Design review of the part built by this model. Coordinates are the model's own, in mm. Face numbers are marked on the shaded views. Coordinates: 2 decimals unless noted, no trailing zeros. Write each loop counter-clockwise with the first axis right and the second up, starting at its lowest first coordinate (ties: lowest second). Pieces come first, ordered by that corner, then holes. Notation, with made-up numbers: M -9.75,51 L 35.25,51 A24 ccw 35.25,81 Z; hole C 14,24.25 d4. An arc over 180 degrees is marked long. Return JSON: item names as keys, results as strings. Group by question number.
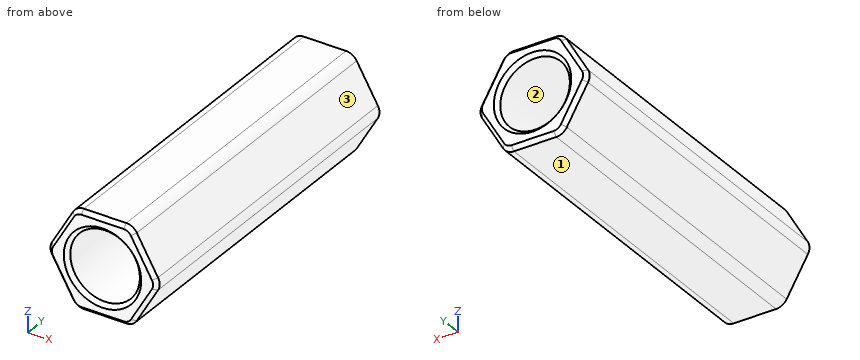
```python
from build123d import *

# Parameters (mm, degrees)
BOSS_EXTRUDE1_DEPTH   = 5.55625
F_4_40_TAPPED_HOLE1_D = 2.2606
FILLET1_R             = 0.396875
CHAMFER1_SIZE         = 0.127


with BuildPart() as part:
    # Sketch1 → Boss-Extrude1 (new body, symmetric)
    with BuildSketch(Plane(origin=(0, 0, 0), x_dir=(1, 0, 0), z_dir=(0, 1, 0))):
        Polygon((0.916543552, 1.5875), (-0.916543552, 1.5875), (-1.833087105, 0), (-0.916543552, -1.5875), (0.916543552, -1.5875), (1.833087105, 0), align=None)
    extrude(amount=BOSS_EXTRUDE1_DEPTH, both=True)

    # #4-40 Tapped Hole1 (through all)
    with Locations(Plane(origin=(0, 5.55625, 0), x_dir=(1, 0, 0), z_dir=(0, 1, 0))):
        with Locations((0, 0)):
            Hole(F_4_40_TAPPED_HOLE1_D / 2)

    # Fillet1
    fillet1_edges = [part.edges().sort_by_distance(p)[0] for p in [
        (1.833087105, 0, 0),
        (0.916543552, 0, 1.5875),
        (-0.916543552, 0, 1.5875),
        (-1.833087105, 0, 0),
        (-0.916543552, 0, -1.5875),
        (0.916543552, 0, -1.5875),
    ]]
    fillet(fillet1_edges, radius=FILLET1_R)

    # Chamfer1
    chamfer1_edges = [part.edges().sort_by_distance(p)[0] for p in [
        (1.1303, 5.55625, 0),
        (1.1303, -5.55625, 0),
        (-1.374815329, -5.55625, -0.79375),
        (-1.374815329, 5.55625, -0.79375),
        (1.374815329, -5.55625, -0.79375),
        (1.374815329, -5.55625, 0.79375),
        (0, -5.55625, 1.5875),
        (-1.374815329, -5.55625, 0.79375),
        (0, -5.55625, -1.5875),
        (-1.771690329, -5.55625, 0),
        (-0.885845164, -5.55625, 1.534328832),
        (0.885845164, -5.55625, 1.534328832),
        (1.771690329, -5.55625, 0),
        (0.885845164, -5.55625, -1.534328832),
        (-0.885845164, -5.55625, -1.534328832),
        (0, 5.55625, -1.5875),
        (1.374815329, 5.55625, -0.79375),
        (-1.374815329, 5.55625, 0.79375),
        (0, 5.55625, 1.5875),
        (1.374815329, 5.55625, 0.79375),
        (-1.771690329, 5.55625, 0),
        (-0.885845164, 5.55625, 1.534328832),
        (0.885845164, 5.55625, 1.534328832),
        (1.771690329, 5.55625, 0),
        (0.885845164, 5.55625, -1.534328832),
        (-0.885845164, 5.55625, -1.534328832),
    ]]
    chamfer(chamfer1_edges, length=CHAMFER1_SIZE)


solid = part.part
```
Item 1: The part is to be moulded in two halves that separate along Z. For the marked faces 1, 2 and 3, say which applies: pulls with the +Z half, pulls with the -Z half, needs draft (parallel to the pull), parting line crosses it, or undercut.
Item 2: Add section C-C (z = 0). Write out the cut boundary in (x, y).
Item 3: Add section A-A (x = 0). Write out the cut boundary in (y, z), plus the area to 3 significant figures.
Item 4: For pin 1 (1.5 mm diameter, centred on y = -4, z = 0.5, fed in from +X); pin 2 (1.5 mm diameter, centred on y = 1, z = -1, fed in from +X), all flat-tipped, find the tip position at first contact; note any pin that passes through.
Item 5: For line 1 (X direction, y = 0, z = 0); line 2 (Z direction, x = 0, y = -1); line 3 (X direction, y = 2.25, z = -0.9), list the stretches that pass through material, from the lowest coordinate up.
Item 6: Add section B-B (y = 1.75). Write out the cut boundary in (x, z), plus the area to 3 significant figures.
Geometry check:
{
 "1": {"face 1": "pulls with the -Z half", "face 2": "undercut", "face 3": "pulls with the +Z half"},
 "2": {"outline": "M -1.77,-5.43 L -1.64,-5.56 L -1.26,-5.56 L -1.13,-5.43 L -1.13,5.43 L -1.26,5.56 L -1.64,5.56 L -1.77,5.43 Z; M 1.13,-5.43 L 1.26,-5.56 L 1.64,-5.56 L 1.77,-5.43 L 1.77,5.43 L 1.64,5.56 L 1.26,5.56 L 1.13,5.43 Z"},
 "3": {"outline": "M -5.56,-1.46 L -5.43,-1.59 L 5.43,-1.59 L 5.56,-1.46 L 5.56,-1.26 L 5.43,-1.13 L -5.43,-1.13 L -5.56,-1.26 Z; M -5.56,1.26 L -5.43,1.13 L 5.43,1.13 L 5.56,1.26 L 5.56,1.46 L 5.43,1.59 L -5.43,1.59 L -5.56,1.46 Z", "area": "10.1 mm^2"},
 "4": {"pin 1": "x = 1.77", "pin 2": "x = 1.69"},
 "5": {"line 1": "-1.77 to -1.13, 1.13 to 1.77", "line 2": "-1.59 to -1.13, 1.13 to 1.59", "line 3": "-1.31 to -0.68, 0.68 to 1.31"},
 "6": {"outline": "M -1.72,-0.2 L -1.03,-1.39 A0.4 ccw -0.69,-1.59 L 0.69,-1.59 A0.4 ccw 1.03,-1.39 L 1.72,-0.2 A0.4 ccw 1.72,0.2 L 1.03,1.39 A0.4 ccw 0.69,1.59 L -0.69,1.59 A0.4 ccw -1.03,1.39 L -1.72,0.2 A0.4 ccw Z; hole C 0,0 d2.26", "area": "4.67 mm^2"}
}
